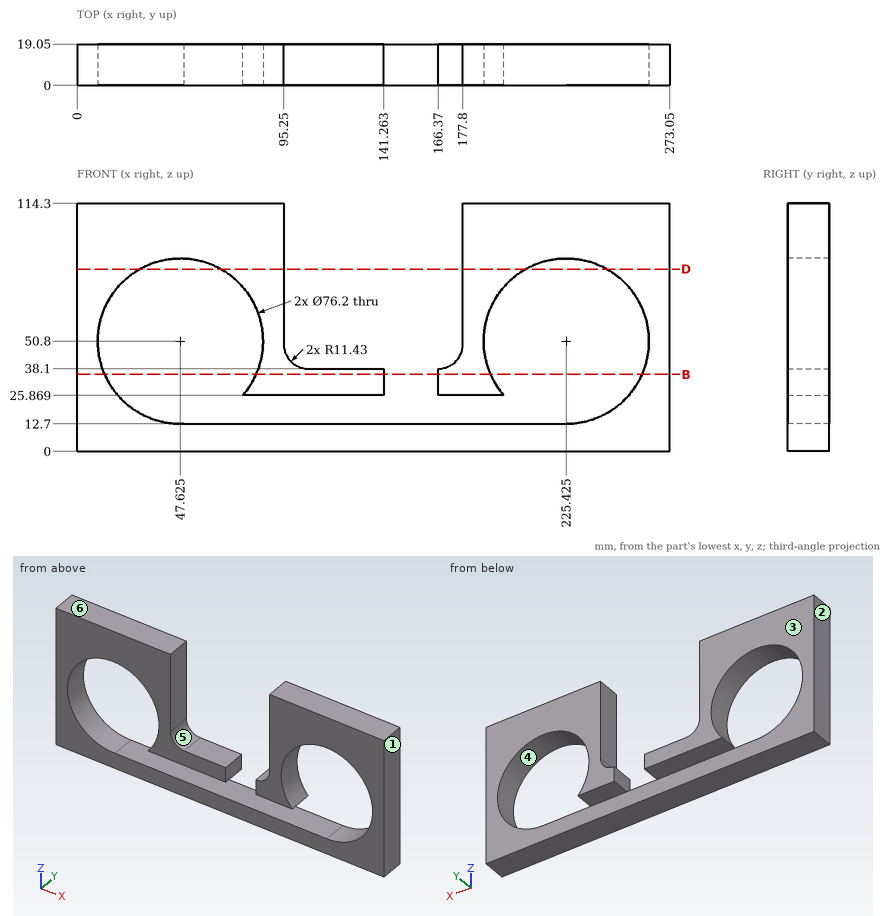
Verification items for this drawing (mm, ordinates from the low corner). A direction names the side the tool comes from. Round coordinates to 2 decimals unless told otherwise and drop trailing zeros. Order: outer loops, then holes, each group sorted by start corner. A loop starts at its lowest first (then second) coordinate and runs counter-clockwise, first axis right, second up. Notation, with made-up numbers: M -30,47.5 L -18,47.5 A28 cw -18,74.5 Z; hole C 42,78.5 d6. An arc over 180 degrees is marked long. Answer in a Markdown table with one row per item. Add a question column.
Item 1: Set-up check for the marked faces 5 and 6: record each of +Z, -Z, +X, -X, +Y, -Y from which the full face is reachable in a straight line by a thin tool's end or side.
Item 2: Sectioned sample at D-D, the plane z = 84. Enter the section's corners in (x, y).
Item 3: Sectioned sample at B-B, the plane z = 35.5. Enter the section's corners in (x, y), plus the area to 3 significant figures.
Item 4: Depth check by flat-ended pin: pin 1 Ø6 at (x, y) = (150, 16.5) entering from +Z; pin 2 Ø5.5 at (x, y) = (121, 9.5) entering from +Z. Enter the tip coordinate at first touch or a pass-through.
Item 5: Draft check along X on the marked faces 1, 2, 3 and 4. Enter one of: released by +X, released by -X, zero draft, split by the parting line, or undercut.
Item 6: Material ranges on L1, parallel to X at y = 4.75, z = 104; L2, parallel to X at y = 18.25, z = 42.5; L3, parallel to Z at x = 185, y = 17.5, recorded low to high. Write a range as [from, to].
Filled in:
| question | item | result |
|---|---|---|
| 1 | face 5 | +Z, +Y, -Y |
| 1 | face 6 | +Z, +X, -X, +Y, -Y |
| 2 | outline | M 0,0 L 28.93,0 L 28.93,19.05 L 0,19.05 Z; M 66.32,0 L 95.25,0 L 95.25,19.05 L 66.32,19.05 Z; M 177.8,0 L 206.73,0 L 206.73,19.05 L 177.8,19.05 Z; M 244.12,0 L 273.05,0 L 273.05,19.05 L 244.12,19.05 Z |
| 3 | outline | M 0,0 L 12.73,0 L 12.73,19.05 L 0,19.05 Z; M 82.52,0 L 141.26,0 L 141.26,19.05 L 82.52,19.05 Z; M 166.37,0 L 190.53,0 L 190.53,19.05 L 166.37,19.05 Z; M 260.32,0 L 273.05,0 L 273.05,19.05 L 260.32,19.05 Z |
| 3 | area | 2,060 mm² |
| 4 | pin 1 | stops at z = 12.71 |
| 4 | pin 2 | stops at z = 38.1 |
| 5 | face 1 | released by +X |
| 5 | face 2 | released by -X |
| 5 | face 3 | zero draft |
| 5 | face 4 | undercut |
| 6 | L1 | x = [0, 95.25], [177.8, 273.05] |
| 6 | L2 | x = [0, 10.44], [84.81, 97.67], [175.38, 188.24], [262.61, 273.05] |
| 6 | L3 | z = [0, 12.71], [25.87, 114.3] |
